```python
from build123d import *

# Parameters (mm, degrees)
F3_FACE_R   = 9.96
F3_FACE_R_2 = 7.96
F2_DEPTH    = 9.751


with BuildPart() as f3:
    # F0 (on Front) → F3 (revolve)
    with BuildSketch(Plane.XZ):
        with BuildLine():
            ThreePointArc((0, 12.5), (-8.8388347648, 8.8388347648), (-12.5, 0))
            Line((-12.5, 0), (-9.96, 0))
            Line((-9.96, 0), (-9.96, -4.25))
            Line((-9.96, -4.25), (-10.96, -4.25))
            Line((-10.96, -4.25), (-9.96, -9.75))
            Line((-9.96, -9.75), (-7.96, -9.75))
            Line((-7.96, -9.75), (-7.96, 0))
            ThreePointArc((-7.96, 0), (-5.6285699782, 5.6285699782), (0, 7.96))
            Line((0, 7.96), (0, 12.5))
        make_face()
    revolve(axis=Axis((0, 0, 10.23), (0, 0, -1)))

    # F1 (on Top) + F3_face (on face) → F2 (cut, through all)
    with BuildSketch(Plane.XY):
        Polygon((1.712546451, 2.9807411881), (1.712546451, 21.5978231281), (-1.712546451, 21.5978231281), (-1.712546451, 2.9374864114), (-0.0125165538, 1.9750342288), align=None)
        Polygon((17.7959412298, 12.3573158479), (1.712546451, 2.9807411881), (1.712546451, 0.998409843), (3.4376094559, 0.0217854573), (19.5210042346, 9.3983601171), align=None)
        Polygon((1.712546451, 0.998409843), (1.712546451, 2.9807411881), (-0.0125165538, 1.9750342288), align=None)
        Polygon((-0.0125165538, 1.9750342288), (-1.712546451, 2.9374864114), (-1.712546451, 0.983921502), align=None)
        Polygon((-1.712546451, 0.983921502), (-1.712546451, 2.9374864114), (-17.9511316948, 12.1307728565), (-19.6385535579, 9.1501908926), (-3.4376094559, -0.0217854573), align=None)
        Polygon((3.4376094559, 0.0217854573), (1.712546451, 0.998409843), (1.712546451, -0.983921502), align=None)
        Polygon((-1.712546451, -0.998409843), (-1.712546451, 0.983921502), (-3.4376094559, -0.0217854573), align=None)
        Polygon((3.4376094559, 0.0217854573), (1.712546451, -0.983921502), (1.712546451, -2.9374864114), (17.9511316948, -12.1307728565), (19.6385535579, -9.1501908926), align=None)
        Polygon((1.712546451, -2.9374864114), (1.712546451, -0.983921502), (0.0125165538, -1.9750342288), align=None)
        Polygon((0.0125165538, -1.9750342288), (-1.712546451, -0.998409843), (-1.712546451, -2.9807411881), align=None)
        Polygon((-1.712546451, -2.9807411881), (-1.712546451, -0.998409843), (-3.4376094559, -0.0217854573), (-19.5210042346, -9.3983601171), (-17.7959412298, -12.3573158479), align=None)
        Polygon((1.712546451, -21.5978231281), (1.712546451, -2.9374864114), (0.0125165538, -1.9750342288), (-1.712546451, -2.9807411881), (-1.712546451, -21.5978231281), align=None)
    with BuildSketch(Plane(origin=(0, 0, -9.75), x_dir=(1, 0, 0), z_dir=(0, 0, -1))):
        Circle(F3_FACE_R)
        Circle(F3_FACE_R_2, mode=Mode.SUBTRACT)
    extrude(amount=-F2_DEPTH, dir=(0, 0, 1), mode=Mode.SUBTRACT)


solid = f3.part
```
The model under review builds one solid part; all positions refer to its coordinate system, in mm. A direction names the side the tool comes from. Give positions to 0.01 mm unless a question says otherwise; leave off trailing zeros. Loops run counter-clockwise (first coordinate to the right, second up) from the corner with the lowest first, then second, coordinate; pieces in that order, holes last. Notation, with made-up numbers: (-1, 61) - (53, 61) arc R25 ccw to (53, 84) - close; hole circle Ø2 at (0.25, 34.25). An arc over 180 degrees is marked (long way). Answer as a JSON object with one key per item and string values.
Q1. To check wall thickness, follow line 1 along X through (y, z) = (-8.25, 5.5); line 2 along Y through (x, z) = (7.5, -1.25); line 3 along Y through (x, z) = (4, 5.75). State the ranges of each line that lie inside material, in increasing order.
Worked out:
{"line 1": "x = -7.61 to 7.61", "line 2": "y = -6.55 to -6.21, 6.35 to 6.55", "line 3": "y = -10.35 to -3.78, 3.78 to 10.35"}
Q2. Add section A-A on z = -6.75. State the section outline as (x, y) points, plus the area to 3 significant figures.
Worked out:
{"outline": "(-9.86, 3.62) arc R10.51 ccw to (-9.82, -3.74) - (-7.58, -2.44) arc R7.96 cw to (-7.61, 2.34) - close; (-8.18, 6.6) - (-5.92, 5.32) arc R7.96 cw to (-1.71, 7.77) - (-1.71, 10.36) arc R10.51 ccw to start; (-8.09, -6.7) arc R10.51 ccw to (-1.71, -10.36) - (-1.71, -7.77) arc R7.96 cw to (-5.85, -5.39) - close; (1.71, -10.36) arc R10.51 ccw to (8.18, -6.6) - (5.92, -5.32) arc R7.96 cw to (1.71, -7.77) - close; (1.71, 7.77) arc R7.96 cw to (5.85, 5.39) - (8.09, 6.7) arc R10.51 ccw to (1.71, 10.36) - close; (7.58, 2.44) arc R7.96 cw to (7.61, -2.34) - (9.86, -3.62) arc R10.51 ccw to (9.82, 3.74) - close", "area": "95.0 mm^2"}
Q3. Add section C-C on x = 1. State the section outline as (y, z) points.
Worked out:
{"outline": "(-12.46, 0) - (-7.9, 0) arc R7.9 cw to (7.9, 0) - (12.46, 0) arc R12.46 ccw to start"}
Q4. Insertion check: pin 1 (4 mm diameter, centred on y = 2.5, z = -2.5, fed in from +X); pin 2 (1.5 mm diameter, centred on y = 9, z = -3, fed in from -X); pin 3 (2.5 mm diameter, centred on x = -5, y = 9, fed in from +Z). Each pin has a flat end and moves straight along its axis. Give the tip position at first contact, or say it passes through.
Worked out:
{"pin 1": "stops at x = 10.85", "pin 2": "stops at x = -5.58", "pin 3": "stops at z = 8.63"}
Q5. For faces 1 (the cylindrical face through (-4.04, 6.86, -4.81)), 2 (the cylindrical face through (-9.96, -0.11, -2.15)), 3 (the flat face through (-6.935, 5.894, -4.807)), 4 (the flat face through (0.2, -8.2, 0)), 5 (the cylindrical face through (-5.06, 8.58, -2.15)), list the 3-axis set-ups (+Z, -Z, +X, -X, +Y, -Y) from which the entire face can be reached by the end or side of a thin tool; tool diameter is ignored.
Worked out:
{"face 1": "-Z", "face 2": "-X", "face 3": "-Z, -X", "face 4": "none", "face 5": "-X, +Y"}
Q6. Add section B-B on y = -10.25. Count the separate pieces of the cut face and the enclosed holes in it, plus the area to 3 significant figures.
Worked out:
{"separate pieces": "3", "enclosed holes": "0", "area": "88.0 mm^2"}
Q7. Add section D-D on z = 10.25. State the section outline as (x, y) points, plus the area to 3 significant figures.
Worked out:
{"outline": "circle Ø14.31 at (0, 0)", "area": "161 mm^2"}
Q8. Mouldability with a two-part tool opening along Y and no side actions: class faces 6 (the flat face through (5, 9, -4.25)), 7 (the flat face through (-6.897, -6.003, -4.807)), 8 (the conical face through (5.16, 9.09, -7.04)) as +Y half, -Y half, draft (parallel to the pull), parting line (faces both ways), or undercut.
Worked out:
{"face 6": "draft", "face 7": "undercut", "face 8": "+Y half"}
